Here's how the part is built. I have some questions about the finished solid (model axes, mm). A direction names the side the tool comes from. Round coordinates to 2 decimals unless told otherwise and drop trailing zeros. Write each loop counter-clockwise with the first axis right and the second up, starting at its lowest first coordinate (ties: lowest second). Pieces come first, ordered by that corner, then holes. Notation, with made-up numbers: (6, 86) -> (26, 86) arc R25 cw to (26, 122) -> close; hole circle Ø1 at (-16, -38). An arc over 180 degrees is marked (long way). Answer as CSV lines item,"result".
from build123d import *

# Parameters (mm, degrees)
F1_DEPTH = 63.5
F2_DEPTH = 25.4
F3_DEPTH = 7.9375
F5_R     = 6.35


with BuildPart() as f1:
    # F0 (on Front) → F1 (new body, symmetric)
    with BuildSketch(Plane.XZ):
        Polygon((-41.275, -9.525), (41.275, -9.525), (41.275, 9.525), (22.225, 9.525), (-41.275, 9.525), align=None)
    extrude(amount=F1_DEPTH, both=True)

    # F0 (on Front) → F2 (join, symmetric)
    with BuildSketch(Plane.XZ):
        with BuildLine():
            Line((22.225, 9.525), (41.275, 9.525))
            Line((41.275, 9.525), (41.275, 38.1))
            ThreePointArc((41.275, 38.1), (47.109768429, 50.3967221242), (60.325, 53.6542598667))
            Line((60.325, 53.6542598667), (60.325, 60.8617413577))
            add(Edge.make_bspline(
                [(27.1694495599, 56.0143021161), (38.4463876666, 58.5668881117), (49.8029060686, 60.022138531), (60.325, 60.8617413577)],
                knots=[78.5242181533, 78.5242181533, 78.5242181533, 78.5242181533, 110.2246687144, 110.2246687144, 110.2246687144, 110.2246687144], degree=3))
            ThreePointArc((27.1694495599, 56.0143021161), (23.4837977408, 47.3920638418), (22.225, 38.1))
            Line((22.225, 38.1), (22.225, 9.525))
        make_face()
        with BuildLine():
            ThreePointArc((77.2304631421, 66.675), (49.8756923374, 72.2590408681), (27.1694495599, 56.0143021161))
            add(Edge.make_bspline(
                [(27.1694495599, 56.0143021161), (38.4463876666, 58.5668881117), (49.8029060686, 60.022138531), (60.325, 60.8617413577)],
                knots=[78.5242181533, 78.5242181533, 78.5242181533, 78.5242181533, 110.2246687144, 110.2246687144, 110.2246687144, 110.2246687144], degree=3))
            Line((60.325, 60.8617413577), (60.325, 66.675))
            Line((60.325, 66.675), (77.2304631421, 66.675))
        make_face()
        with BuildLine():
            Line((60.325, 60.8617413577), (60.325, 53.6542598667))
            ThreePointArc((60.325, 53.6542598667), (67.7756703476, 49.8945222313), (72.2897850038, 42.8752))
            Line((72.2897850038, 42.8752), (85.725, 42.8752))
            Line((85.725, 42.8752), (85.725, 61.9252))
            Line((85.725, 61.9252), (82.6865516458, 61.9252))
            add(Edge.make_bspline(
                [(60.325, 60.8617413577), (68.4096639512, 61.5068512332), (76.0017140406, 61.7885051595), (82.6865516458, 61.9252)],
                knots=[110.2246687144, 110.2246687144, 110.2246687144, 110.2246687144, 134.5817493068, 134.5817493068, 134.5817493068, 134.5817493068], degree=3))
        make_face()
        with BuildLine():
            ThreePointArc((82.6865516458, 61.9252), (80.0818154438, 64.4417437815), (77.2304631421, 66.675))
            Line((77.2304631421, 66.675), (60.325, 66.675))
            Line((60.325, 66.675), (60.325, 60.8617413577))
            add(Edge.make_bspline(
                [(60.325, 60.8617413577), (68.4096639512, 61.5068512332), (76.0017140406, 61.7885051595), (82.6865516458, 61.9252)],
                knots=[110.2246687144, 110.2246687144, 110.2246687144, 110.2246687144, 134.5817493068, 134.5817493068, 134.5817493068, 134.5817493068], degree=3))
        make_face()
    extrude(amount=F2_DEPTH, both=True)

    # F0 (on Front) → F3 (join, symmetric)
    with BuildSketch(Plane.XZ):
        with BuildLine():
            add(Edge.make_bspline(
                [(-41.275, 9.525), (-28.2097739582, 36.6353245675), (-0.7643094977, 49.6913692863), (27.1694495599, 56.0143021161)],
                knots=[0, 0, 0, 0, 78.5242181533, 78.5242181533, 78.5242181533, 78.5242181533], degree=3))
            Line((-41.275, 9.525), (22.225, 9.525))
            Line((22.225, 9.525), (22.225, 38.1))
            ThreePointArc((22.225, 38.1), (23.4837977408, 47.3920638418), (27.1694495599, 56.0143021161))
        make_face()
    extrude(amount=F3_DEPTH, both=True)

    # F0 (on Front) → F4 (revolve)
    with BuildSketch(Plane.XZ):
        Polygon((111.125, 66.675), (85.725, 66.675), (85.725, 61.9252), (85.725, 42.8752), (85.725, 38.1), (111.125, 38.1), align=None)
    revolve(axis=Axis((85.725, 0, 52.3875), (0, 0, 1)))

    # F5
    f5_edges = [f1.edges().sort_by_distance(p)[0] for p in [
        (41.275, -63.5, 0),
        (41.275, 63.5, 0),
        (-41.275, 63.5, 0),
        (-41.275, -63.5, 0),
    ]]
    fillet(f5_edges, radius=F5_R)


solid = f1.part
Item 1: Suppose I cut it at B-B, the plane y = -48. List the corners of the cut face in (x, z) for me (3 decimals), then the cut area to 3 significant figures.
Results found:
outline,"(-41.275, -9.525) -> (41.275, -9.525) -> (41.275, 9.525) -> (-41.275, 9.525) -> close"
area,"1,570 mm²"
Item 2: Suppose I cut it at C-C, the plane x = 95. List the corners of the cut face in (y, z) for me (3 decimals), then the cut area to 3 significant figures.
Results found:
outline,"(-23.646, 38.1) -> (23.646, 38.1) -> (23.646, 66.675) -> (-23.646, 66.675) -> close"
area,"1,350 mm²"
Item 3: If we mould it in two halves opening along X, with no side actions, what happens to faces 5 (the cylindrical face through (-39.464, -61.59, -0.133)), 6 (the flat face through (86, 0, 38.1)), 7 (the flat face through (75, -24, 42.875))? For each: pulls with the +X half, pulls with the -X half, needs draft (parallel to the pull), parting line crosses it, or undercut.
Results found:
face 5,"pulls with the -X half"
face 6,"needs draft"
face 7,"undercut"
Item 4: Suppose I cut it at A-A, the plane x = 67.5. List the corners of the cut face in (y, z) for me.
Results found:
outline,"(-25.4, 50.14) -> (-17.69, 50.14) -> (-17.69, 38.1) -> (17.69, 38.1) -> (17.69, 50.14) -> (25.4, 50.14) -> (25.4, 71.46) -> (-25.4, 71.46) -> close"
Item 5: For faces 1 (the flat face through (-7, -7.938, 28)), 2 (the flat face through (-7, 7.938, 28)), 3 (the flat face through (39, 25.4, 49)), 4 (the flat face through (39, -25.4, 49)), which set-ups out of +Z, -Z, +X, -X, +Y, -Y let a thin tool reach every point of the face, with its end or its side?
Results found:
face 1,"+Z, -X, -Y"
face 2,"+Z, -X, +Y"
face 3,"+Z, +X, -X, +Y"
face 4,"+Z, +X, -X, -Y"
Item 6: Will these pins go through, and if not, where does the flat tip stop? pin 1 (6 mm diameter, centred on x = 54, z = 54.5, fed in from -Y); pin 2 (1.9 mm diameter, centred on x = 79.5, y = -23, fed in from -Z); pin 3 (23 mm diameter, centred on x = -8.5, z = 22, fed in from -Y).
Results found:
pin 1,"stops at y = -25.4"
pin 2,"stops at z = 38.1"
pin 3,"stops at y = -7.94"
Item 7: I need wall thicknesses on L1, parallel to Z at x = -0.5, y = -11 (3 decimals); L2, parallel to X at y = 14, z = 5 (3 decimals); L3, parallel to Y at x = -16.5, z = 24. Which ranges of each line are inside material? Lowest first, please.
Results found:
L1,"z = -9.525 to 9.525"
L2,"x = -41.275 to 41.275"
L3,"y = -7.94 to 7.94"
